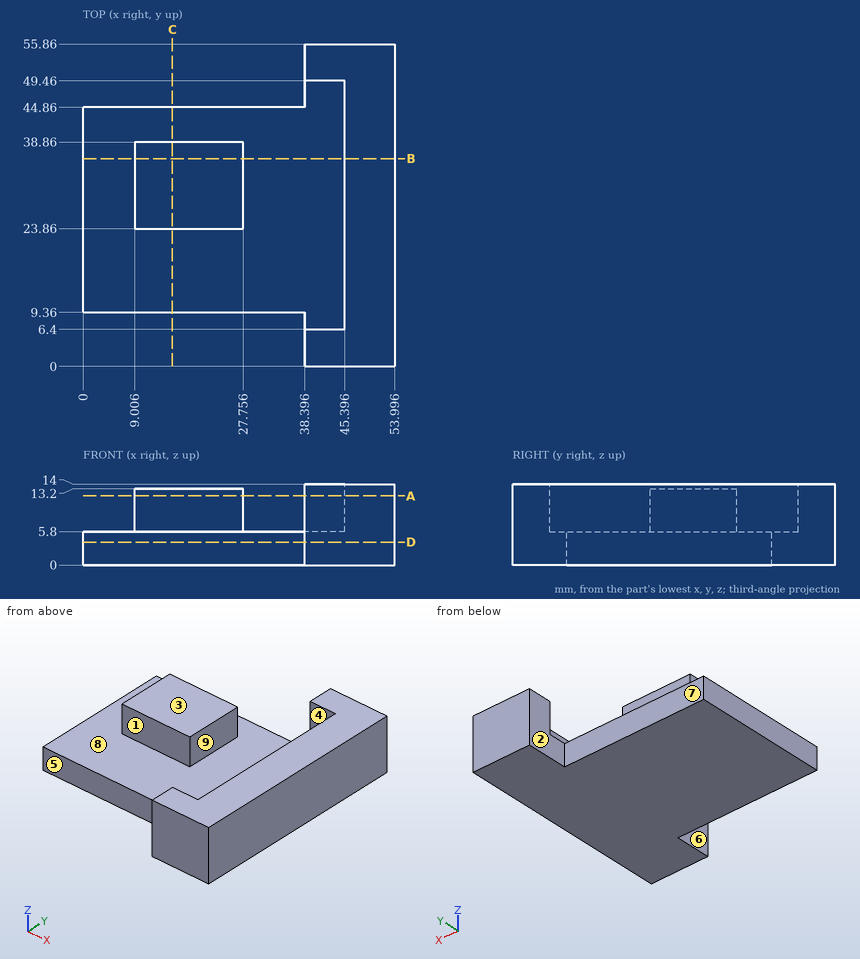
Print and shaded views of the part. All mm, measured from the part's lowest x, y and z. A direction names the side the tool comes from. Coordinates: 2 decimals unless noted, no trailing zeros. Order: outer loops, then holes, each group sorted by start corner. A loop starts at its lowest first (then second) coordinate and runs counter-clockwise, first axis right, second up. Notation, with made-up numbers: M -23,-3.5 L 9,-3.5 A15 ccw 9,25.5 Z; hole C -15,86.5 d1. An arc over 180 degrees is marked long. Write each question's results on one line, items separated by ' | '. Start each with the question number.
Q1. Cut at C-C (x = 15.5). List the corners of the cut face in (y, z).
Q2. Cut at D-D (z = 4). List the corners of the cut face in (x, y).
Q3. Cut at B-B (y = 36). List the corners of the cut face in (x, z).
Q4. Pull direction X, two halves, no side cores. Call the marked faces 6, 7, 8 and 9: +X half, -X half, draft (parallel to the pull), parting line (faces both ways), or undercut.
Q5. Cut at A-A (z = 12). List the corners of the cut face in (x, y), then the cut area to 3 significant figures.
Q6. Flat gauge pins, fed straight in: P1, Ø3, axis at y = 24.5, z = 6.5, coming from the -X side; P2, Ø2.5, axis at y = 30.5, z = 11.5, coming from the -X side; P3, Ø2, axis at x = 22, z = 11.5, coming from the -Y side; P4, Ø2, axis at x = 19.5, z = 10, coming from the +Y side. Where does each tip first touch, or does it go through?
Q7. Drill centre lines: probe 1 along X at (y, z) = (27, 12.5); probe 2 along Y at (x, z) = (41, 13.5); probe 3 along Y at (x, z) = (18, 4.25). Where is each one in solid material? Low to high. Write a range as from..to.
Q8. Which spindle directions (+Z, -Z, +X, -X, +Y, -Y) get a long thin tool onto all of the face, cutting with end or side? Do the marked faces 1, 2, 3, 4 and 5. Say none if no direction does.
Found:
1) outline: M 9.36,0 L 44.86,0 L 44.86,5.8 L 38.86,5.8 L 38.86,13.2 L 23.86,13.2 L 23.86,5.8 L 9.36,5.8 Z
2) outline: M 0,9.36 L 38.4,9.36 L 38.4,0 L 54,0 L 54,55.86 L 38.4,55.86 L 38.4,44.86 L 0,44.86 Z
3) outline: M 0,0 L 54,0 L 54,14 L 45.4,14 L 45.4,5.8 L 27.76,5.8 L 27.76,13.2 L 9.01,13.2 L 9.01,5.8 L 0,5.8 Z
4) face 6: -X half | face 7: draft | face 8: undercut | face 9: undercut
5) outline: M 9.01,23.86 L 27.76,23.86 L 27.76,38.86 L 9.01,38.86 Z; M 38.4,0 L 54,0 L 54,55.86 L 38.4,55.86 L 38.4,49.46 L 45.4,49.46 L 45.4,6.4 L 38.4,6.4 Z | area: 851 mm²
6) P1: x = 0 | P2: x = 9.01 | P3: y = 23.86 | P4: y = 38.86
7) probe 1: 9.01..27.76, 45.4..54 | probe 2: 0..6.4, 49.46..55.86 | probe 3: 9.36..44.86
8) face 1: +Z, -X, -Y | face 2: +Z, -Z, -X, +Y | face 3: +Z, -X, +Y, -Y | face 4: +Z, -X | face 5: +Z, -Z, -X, -Y
